Design review of the part built by this model. Coordinates are the model's own, in mm. Face numbers are marked on the shaded views. Give positions to 0.01 mm unless a question says otherwise; leave off trailing zeros. Loops run counter-clockwise (first coordinate to the right, second up) from the corner with the lowest first, then second, coordinate; pieces in that order, holes last. Notation, with made-up numbers: (89, -13) - (118, -13) arc R12 ccw to (118, 0) - close; hole circle Ø11 at (8.5, 17). An arc over 180 degrees is marked (long way). Write each question's results on one line, items separated by ' | '.
from build123d import *

# Parameters (mm, degrees)
SKETCH1_W           = 100
SKETCH1_H           = 100
BASE_DEPTH          = 10
SKETCH2_R           = 10.5
LOAD_CELL_CUT_DEPTH = 1
CUT_EXTRUDE1_REACH  = 73.414
SKETCH15_R          = 3
SKETCH21_R          = 2.5
CUT_EXTRUDE2_DEPTH  = 10


with BuildPart() as part:
    # Sketch1 → base (new body)
    with BuildSketch(Plane(origin=(0, 0, 0), x_dir=(1, 0, 0), z_dir=(0, 1, 0))):
        Rectangle(SKETCH1_W, SKETCH1_H)
    extrude(amount=BASE_DEPTH)

    # Sketch2 → load cell cut (cut)
    with BuildSketch(Plane(origin=(0, 10, 0), x_dir=(1, 0, 0), z_dir=(0, 1, 0))):
        with Locations(Location((0, 0, 0), (0, 0, 270))):
            Circle(SKETCH2_R)
    extrude(amount=-LOAD_CELL_CUT_DEPTH, mode=Mode.SUBTRACT)

    # Sketch15 → Cut-Extrude1 (cut, up to next)
    with BuildSketch(Plane(origin=(0, 0, 0), x_dir=(-1, 0, 0), z_dir=(0, -1, 0)), mode=Mode.PRIVATE) as cut_extrude1_sk1:
        with Locations(Location((40, -40, 0), (0, 0, 90))):
            Circle(SKETCH15_R)
    cut_extrude1_tool1 = extrude(cut_extrude1_sk1.sketch, amount=-CUT_EXTRUDE1_REACH, mode=Mode.PRIVATE) & part.part
    # Sketch15 → Cut-Extrude1 (cut, up to next)
    with BuildSketch(Plane(origin=(0, 0, 0), x_dir=(-1, 0, 0), z_dir=(0, -1, 0)), mode=Mode.PRIVATE) as cut_extrude1_sk2:
        with Locations(Location((-40, -40, 0), (0, 0, 90))):
            Circle(SKETCH15_R)
    cut_extrude1_tool2 = extrude(cut_extrude1_sk2.sketch, amount=-CUT_EXTRUDE1_REACH, mode=Mode.PRIVATE) & part.part
    # Sketch15 → Cut-Extrude1 (cut, up to next)
    with BuildSketch(Plane(origin=(0, 0, 0), x_dir=(-1, 0, 0), z_dir=(0, -1, 0)), mode=Mode.PRIVATE) as cut_extrude1_sk3:
        with Locations(Location((40, 40, 0), (0, 0, 90))):
            Circle(SKETCH15_R)
    cut_extrude1_tool3 = extrude(cut_extrude1_sk3.sketch, amount=-CUT_EXTRUDE1_REACH, mode=Mode.PRIVATE) & part.part
    # Sketch15 → Cut-Extrude1 (cut, up to next)
    with BuildSketch(Plane(origin=(0, 0, 0), x_dir=(-1, 0, 0), z_dir=(0, -1, 0)), mode=Mode.PRIVATE) as cut_extrude1_sk4:
        with Locations(Location((-40, 40, 0), (0, 0, 90))):
            Circle(SKETCH15_R)
    cut_extrude1_tool4 = extrude(cut_extrude1_sk4.sketch, amount=-CUT_EXTRUDE1_REACH, mode=Mode.PRIVATE) & part.part
    add(cut_extrude1_tool1.solids().sort_by_distance((-40, 0, 40))[0], mode=Mode.SUBTRACT)
    add(cut_extrude1_tool2.solids().sort_by_distance((40, 0, 40))[0], mode=Mode.SUBTRACT)
    add(cut_extrude1_tool3.solids().sort_by_distance((-40, 0, -40))[0], mode=Mode.SUBTRACT)
    add(cut_extrude1_tool4.solids().sort_by_distance((40, 0, -40))[0], mode=Mode.SUBTRACT)

    # Sketch21 → Cut-Extrude2 (cut)
    with BuildSketch(Plane(origin=(0, 0, -50), x_dir=(-1, 0, 0), z_dir=(0, 0, -1))):
        with Locations((-10, 5)):
            Circle(SKETCH21_R)
        with Locations((10, 5)):
            Circle(SKETCH21_R)
    cut_extrude2 = extrude(amount=-CUT_EXTRUDE2_DEPTH, mode=Mode.SUBTRACT)

    # Mirror2: Cut-Extrude2 across plane
    add(cut_extrude2.mirror(Plane.XY), mode=Mode.SUBTRACT)


solid = part.part
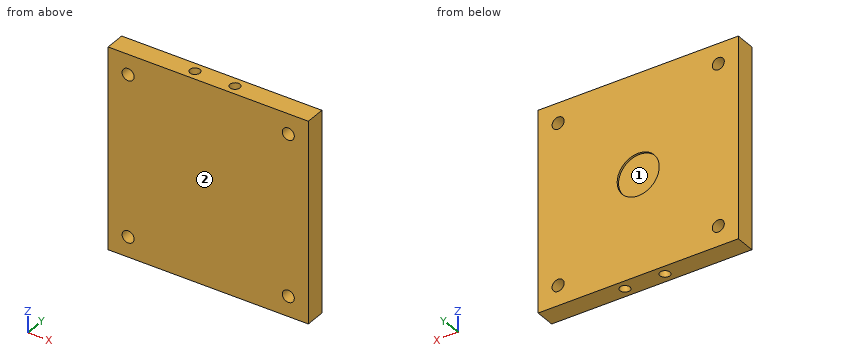
(1) Take a section at D-D on x = -41.5. Give the boundary of the cut face in (y, z).
Answers below:
outline: (0, -50) - (10, -50) - (10, -42.6) - (0, -42.6) - close; (0, -37.4) - (10, -37.4) - (10, 37.4) - (0, 37.4) - close; (0, 42.6) - (10, 42.6) - (10, 50) - (0, 50) - close
(2) Take a section at B-B on y = 5. Give the boundary of the cut face in (x, z).
Answers below:
outline: (-50, -50) - (-12.5, -50) - (-12.5, -40) - (-7.5, -40) - (-7.5, -50) - (7.5, -50) - (7.5, -40) - (12.5, -40) - (12.5, -50) - (50, -50) - (50, 50) - (12.5, 50) - (12.5, 40) - (7.5, 40) - (7.5, 50) - (-7.5, 50) - (-7.5, 40) - (-12.5, 40) - (-12.5, 50) - (-50, 50) - close; hole circle Ø6 at (-40, -40); hole circle Ø6 at (-40, 40); hole circle Ø6 at (40, -40); hole circle Ø6 at (40, 40)
(3) Wall thickness on line 1 along Y through (x, z) = (10, 44.25); line 2 along Z through (x, y) = (-42.5, 9.25); line 3 along X through (y, z) = (9.4, 0): over which ranges is each line inside the solid? List them lowest first. Write a range as from..to.
Answers below:
line 1: 0..2.5, 7.5..10 | line 2: -50..-41.66, -38.34..38.34, 41.66..50 | line 3: -50..-10.5, 10.5..50
(4) Take a section at A-A on x = 40. Give the boundary of the cut face in (y, z), plus the area to 3 significant figures.
Answers below:
outline: (0, -50) - (10, -50) - (10, -43) - (0, -43) - close; (0, -37) - (10, -37) - (10, 37) - (0, 37) - close; (0, 43) - (10, 43) - (10, 50) - (0, 50) - close | area: 880 mm2
(5) Draft analysis for pull direction Z (two halves, no side actions). For the marked faces 1 and 2, state which applies: pulls with the +Z half, pulls with the -Z half, needs draft (parallel to the pull), parting line crosses it, or undercut.
Answers below:
face 1: undercut | face 2: needs draft
(6) Take a section at C-C on z = 0. Give the boundary of the cut face in (x, y).
Answers below:
outline: (-50, 0) - (50, 0) - (50, 10) - (10.5, 10) - (10.5, 9) - (-10.5, 9) - (-10.5, 10) - (-50, 10) - close
(7) Insertion check: P1, Ø3, axis at x = 2, z = -39.5, coming from the -Y side; P2, Ø2.5, axis at x = 10, y = 5.5, coming from the +Z side; P3, Ø6.5, axis at x = 4, z = 0, coming from the +Y side; P4, Ø2.5, axis at x = -11, y = 5, coming from the -Z side. Each pin has a flat end and moves straight along its axis. Give the tip position at first contact, or say it passes through.
Answers below:
P1: y = 0 | P2: z = 40 | P3: y = 9 | P4: z = -40
